Autodesk Inventor part; units mm, degrees
ref_plane "YZ Plane" through (0, 0, 0) normal (1, 0, 0) x (0, 1, 0)
ref_plane "XZ Plane" through (0, 0, 0) normal (0, 1, 0) x (-1, 0, 0)
ref_plane "XY Plane" through (0, 0, 0) normal (0, 0, 1) x (1, 0, 0)
sketch "Boceto3" plane through (0, 0, 0) normal (0, 1, 0) x (-1, 0, 0)
  circle A0 centre (0, 0) radius 5
  dimension "d21" = 10
extrude "Extrusión2" add sketch "Boceto3" along normal blind 180
sketch "Boceto4" plane through (0, 0, 0) normal (0, -1, 0) x (1, 0, 0)
  line L0 (-7.5, -7.5) -> (7.5, -7.5)
  line L1 (7.5, -7.5) -> (7.5, 7.5)
  line L2 (7.5, 7.5) -> (-7.5, 7.5)
  line L3 (-7.5, 7.5) -> (-7.5, -7.5)
  line L4 (-7.5, -7.5) -> (7.5, 7.5) construction
  line L5 (7.5, -7.5) -> (-7.5, 7.5) construction
  point P0 (0, 0)
  dimension "d24" = 15
  dimension "d25" = 15
extrude "Extrusión3" add sketch "Boceto4" along normal blind 15
sketch "Boceto5" plane through (0, -15, 0) normal (0, -1, 0) x (1, 0, 0)
  line L0 (2.5, 6) -> (-2.5, 6)
  line L1 (-2.5, 6) -> (-2.5, -6)
  line L2 (-2.5, -6) -> (2.5, -6)
  line L3 (2.5, -6) -> (2.5, 6)
  line L4 (2.5, 6) -> (-2.5, -6) construction
  line L5 (-2.5, 6) -> (2.5, -6) construction
  point P0 (0, 0)
  dimension "d28" = 5
  dimension "d29" = 12
extrude "Extrusión4" add sketch "Boceto5" along normal blind 20
sketch "Boceto6" plane through (2.5, -15, 6) normal (1, 0, 0) x (0, 0, -1)
  line L0 (12, -20) -> (0, -20)
  line L1 (6, -20) -> (6, -12)
  circle A0 centre (6, -12) radius 3
  point P0 (6, 15)
  dimension "d32" = 8
  dimension "d33" = 6
extrude "Extrusión5" cut sketch "Boceto6" against normal blind 20
properties part number "pendulum" material "Plástico ABS"
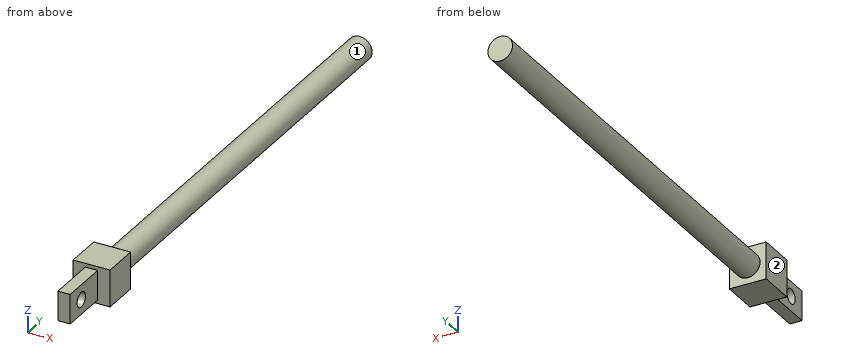
Could you check a few things on this model? Use its own coordinates, in mm. Face numbers are marked on the shaded views. A direction names the side the tool comes from. Give positions to 0.01 mm unless a question says otherwise; leave off trailing zeros. Order: outer loops, then holes, each group sorted by start corner. A loop starts at its lowest first (then second) coordinate and runs counter-clockwise, first axis right, second up. Notation, with made-up numbers: (-26, 31) -> (-4, 31) arc R12 cw to (-4, 36) -> close; hole circle Ø2 at (-11.5, 59). An arc over 180 degrees is marked (long way). Answer in a Markdown table with one row per item. Add a question column.
Item 1: Please list where these lines run through material, in increasing order: probe 1 along Y at (x, z) = (0.75, 0); probe 2 along Z at (x, y) = (0.95, -27); probe 3 along X at (y, z) = (19, -0.25).
Item 2: I'm going to push flat-ended pins straight in: P1, Ø2.5, axis at x = -1, y = -21.5, coming from the -Z side; P2, Ø1.5, axis at x = -4.5, y = 80.5, coming from the +Z side; P3, Ø2, axis at x = -1, y = 43, coming from the -Z side. Where does each tip first touch, or does it pass through?
Item 3: Imagine slicing it at B-B (y = -27). List the corners of the cut face in (x, z) for me, and give its area (3 significant figures).
Item 4: Imagine slicing it at C-C (x = 0). List the corners of the cut face in (y, z) for me.
Item 5: Imagine slicing it at D-D (y = 104). List the corners of the cut face in (x, z) for me.
Item 6: For the marked faces 1 and 2, which set-ups out of +Z, -Z, +X, -X, +Y, -Y let a thin tool reach every point of the face, with its end or its side?
Item 7: Imagine slicing it at A-A (z = 0). List the corners of the cut face in (x, y) for me.
Result:
| question | item | result |
|---|---|---|
| 1 | probe 1 | -35 to -30, -24 to 180 |
| 1 | probe 2 | -6 to -3, 3 to 6 |
| 1 | probe 3 | -4.99 to 4.99 |
| 2 | P1 | z = -6 |
| 2 | P2 | z = 3.31 |
| 2 | P3 | z = -5 |
| 3 | outline | (-2.5, -6) -> (2.5, -6) -> (2.5, -3) -> (-2.5, -3) -> close; (-2.5, 3) -> (2.5, 3) -> (2.5, 6) -> (-2.5, 6) -> close |
| 3 | area | 30.0 mm2 |
| 4 | outline | (-35, -6) -> (-15, -6) -> (-15, -7.5) -> (0, -7.5) -> (0, -5) -> (180, -5) -> (180, 5) -> (0, 5) -> (0, 7.5) -> (-15, 7.5) -> (-15, 6) -> (-35, 6) -> close; hole circle Ø6 at (-27, 0) |
| 5 | outline | circle Ø10 at (0, 0) |
| 6 | face 1 | +Y |
| 6 | face 2 | +Z, -Z, -X, +Y, -Y |
| 7 | outline | (-7.5, -15) -> (-2.5, -15) -> (-2.5, -24) -> (2.5, -24) -> (2.5, -15) -> (7.5, -15) -> (7.5, 0) -> (5, 0) -> (5, 180) -> (-5, 180) -> (-5, 0) -> (-7.5, 0) -> close; (-2.5, -35) -> (2.5, -35) -> (2.5, -30) -> (-2.5, -30) -> close |
